Work out the finished part from the listing and answer in its coordinate system (mm). A direction names the side the tool comes from. Round coordinates to 2 decimals unless told otherwise and drop trailing zeros. Loops run counter-clockwise (first coordinate to the right, second up) from the corner with the lowest first, then second, coordinate; pieces in that order, holes last. Notation, with made-up numbers: (79, -17) -> (98, -17) arc R24 cw to (98, 10) -> close; hole circle Ø11 at (81, 0.5). An arc over 180 degrees is marked (long way). Use CSV: the item, a comma, the result in double quotes. Start each with the question number.
from build123d import *

# Parameters (mm, degrees)
SKETCH1_W      = 35
SKETCH1_H      = 20
EXTRUDE1_DEPTH = 22.5
SKETCH2_R      = 6
EXTRUDE2_DEPTH = 30


with BuildPart() as part:
    # Sketch1 → Extrude1 (new body)
    with BuildSketch(Plane(origin=(0, 0, 0), x_dir=(1, 0, 0), z_dir=(0, 1, 0))):
        with Locations((17.5, 10)):
            Rectangle(SKETCH1_W, SKETCH1_H)
    extrude(amount=-EXTRUDE1_DEPTH)

    # Sketch2 → Extrude2 (add)
    with BuildSketch(Plane(origin=(0, 0, 0), x_dir=(1, 0, 0), z_dir=(0, 1, 0))):
        with Locations(Location((17.5, 10, 0), (0, 0, 270))):  # turned: the seam where the file's is
            Circle(SKETCH2_R)
    extrude(amount=EXTRUDE2_DEPTH)


solid = part.part
Q1. Section C-C, the plane y = 5 is taken. Write down the section's boundary in (x, z).
Q2. Section A-A, the plane z = -10 is taken. Write down the section's boundary in (x, y), and give its area (3 significant figures).
Q3. Which of the six approach directions +Z, -Z, +X, -X, +Y, -Y give full straight-line access (tool end or side, diameter ignored) to faces 1 (the cylindrical face through (19.302, 14.79, -4.277)), 2 (the flat face through (18, 30, -10))?
Q4. Section D-D, the plane x = 32.5 is taken. Write down the section's boundary in (y, z), and give its area (3 significant figures).
Q5. Section B-B, the plane x = 17.5 is taken. Write down the section's boundary in (y, z), and give its area (3 significant figures).
Q6. Each of these flat-tipped pins is pushed along its axis until it touches: pin 1 (10 mm diameter, centred on y = 2, z = -7, fed in from -X); pin 2 (1 mm diameter, centred on y = 14, z = -6.5, fed in from -X); pin 3 (6 mm diameter, centred on y = 17.5, z = -12.5, fed in from -X). Where does it stop, or does it pass through?
Q7. Straight lines are drawn through the part: line 1 (Y direction, x = 8, z = -4); line 2 (Z direction, x = 22, y = 13.5); line 3 (Z direction, x = 23, y = 23.5). For each, find the intervals that lie inside material, in ascending order. Write a range as from..to.
Report:
1,outline,"circle Ø12 at (17.5, -10)"
2,outline,"(0, -22.5) -> (35, -22.5) -> (35, 0) -> (23.5, 0) -> (23.5, 30) -> (11.5, 30) -> (11.5, 0) -> (0, 0) -> close"
2,area,"1,150 mm²"
3,face 1,"+Y"
3,face 2,"+Z, -Z, +X, -X, +Y"
4,outline,"(-22.5, -20) -> (0, -20) -> (0, 0) -> (-22.5, 0) -> close"
4,area,"450 mm²"
5,outline,"(-22.5, -20) -> (0, -20) -> (0, -16) -> (30, -16) -> (30, -4) -> (0, -4) -> (0, 0) -> (-22.5, 0) -> close"
5,area,"810 mm²"
6,pin 1,"stops at x = 0"
6,pin 2,"stops at x = 12.3"
6,pin 3,"stops at x = 11.5"
7,line 1,"y = -22.5..0"
7,line 2,"z = -13.97..-6.03"
7,line 3,"z = -12.4..-7.6"
